from build123d import *

# Parameters (mm, degrees)
F2_R     = 0.508
F3_SIZE  = 6.35
F4_SIZE2 = 3.81
F4_SIZE  = 7.62


with BuildPart() as f1:
    # F0 (on Front) → F1 (revolve)
    with BuildSketch(Plane.XZ):
        Polygon((55.7449534535, 20.7715928555), (0, 20.7715928555), (0, 0), (83.0746293068, 0), (83.0746293068, 26.4260116965), (55.7449534535, 26.4260116965), align=None)
    revolve(axis=Axis((60.4887977242, 0, 0), (1, 0, 0)))

    # F2
    f2_edges = [f1.edges().sort_by_distance(p)[0] for p in [
        (55.744953, 0, -26.426012),
    ]]
    fillet(f2_edges, radius=F2_R)

    # F3
    f3_edges = [f1.edges().sort_by_distance(p)[0] for p in [
        (83.074629, 0, -26.426012),
    ]]
    chamfer(f3_edges, length=F3_SIZE)

    # F4
    f4_edges = [f1.edges().sort_by_distance(p)[0] for p in [
        (0, 0, -20.771593),
    ]]
    f4_side = f1.faces().sort_by_distance((27.872477, 0, -20.771593))[0]
    chamfer(f4_edges, length=F4_SIZE, length2=F4_SIZE2, reference=f4_side)


solid = f1.part
The model under review builds one solid part; all positions refer to its coordinate system, in mm. A direction names the side the tool comes from. Round coordinates to 2 decimals unless told otherwise and drop trailing zeros. Loops run counter-clockwise (first coordinate to the right, second up) from the corner with the lowest first, then second, coordinate; pieces in that order, holes last. Notation, with made-up numbers: (50, 68) -> (109, 68) arc R25 cw to (109, 87) -> close; hole circle Ø11 at (65, 38.5). An arc over 180 degrees is marked (long way). Answer as CSV lines item,"result".
1) Add section A-A on z = 0. Write out the cut boundary in (x, y), plus the area to 3 significant figures.
Geometry results:
outline,"(0, -16.96) -> (7.62, -20.77) -> (55.74, -20.77) -> (55.74, -25.92) arc R0.51 ccw to (56.25, -26.43) -> (76.72, -26.43) -> (83.07, -20.08) -> (83.07, 20.08) -> (76.72, 26.43) -> (56.25, 26.43) arc R0.51 ccw to (55.74, 25.92) -> (55.74, 20.77) -> (7.62, 20.77) -> (0, 16.96) -> close"
area,"3,690 mm²"
2) To check wall thickness, follow line 1 along Z through (x, y) = (36, 12); line 2 along Z through (x, y) = (44.5, -13.5); line 3 along Y through (x, z) = (19.5, -8.5). State the ranges of each line that lie inside material, in increasing order. Write a range as from..to.
Geometry results:
line 1,"z = -16.95..16.95"
line 2,"z = -15.79..15.79"
line 3,"y = -18.95..18.95"
3) Add section D-D on x = 60. Write out the cut boundary in (y, z), plus the area to 3 significant figures.
Geometry results:
outline,"circle Ø52.85 at (0, 0)"
area,"2,190 mm²"
4) For P1, Ø2, axis at x = 34.5, y = 6, coming from the -Z side; P2, Ø2, axis at y = -3.5, z = 4, coming from the -X side; P3, Ø1.5, axis at x = 65, y = -7, coming from the +Z side; P4, Ø2, axis at x = 70.5, z = 3.5, coming from the +Y side, all flat-tipped, find the tip position at first contact; note any pin that passes through.
Geometry results:
P1,"stops at z = -20.16"
P2,"stops at x = 0"
P3,"stops at z = 25.68"
P4,"stops at y = 26.31"
5) Add section C-C on x = 43. Write out the cut boundary in (y, z), plus the area to 3 significant figures.
Geometry results:
outline,"circle Ø41.54 at (0, 0)"
area,"1,360 mm²"
6) Tool access review of faces 1 (the face through (83.075, 0, 0)), 2 (the face through (31.35, 20.28, -4.5)): name each direction out of +Z, -Z, +X, -X, +Y, -Y from which nothing blocks a thin tool from reaching the whole face with its end or side.
Geometry results:
face 1,"+Z, -Z, +X, +Y, -Y"
face 2,"-X"
